CAD build for the part. Positions are in the model's coordinates, mm. A direction names the side the tool comes from. Coordinates: 2 decimals unless noted, no trailing zeros. Order: outer loops, then holes, each group sorted by start corner. A loop starts at its lowest first (then second) coordinate and runs counter-clockwise, first axis right, second up. Notation, with made-up numbers: (-6, 87.5) - (45, 87.5) arc R17 ccw to (45, 92.5) - close; hole circle Ø7 at (7, 53). An arc over 180 degrees is marked (long way). Write each question's results on one line, items separated by ' | '. Start each with the question number.
Q1. Band-saw the part on A-A, the plane z = -95. Write the cut outline in (x, y), then the cut area to 3 significant figures.
Q2. Band-saw the part on D-D, the plane x = -2.5. Write the cut outline in (y, z).
Q3. Pin check, flat tips, straight feed: P1, Ø10, axis at x = -25.5, y = 4.5, coming from the -Z side; P2, Ø4.5, axis at x = 1.5, y = 5.5, coming from the -Z side; P3, Ø1.5, axis at y = 10, z = -56.5, coming from the -X side. Stop position of each tip, or through.
Q4. Wall check: probe 1 along X at (y, z) = (19.75, -8.5); probe 2 along Z at (x, y) = (20, 3); probe 3 along Z at (x, y) = (3.5, 11.75). Give the ranges that are in metal, low to high.
Q5. Which spindle directions (+Z, -Z, +X, -X, +Y, -Y) get a long thin tool onto all of the face, cutting with end or side? Do faces 5 (the flat face through (-31.418, 10.846, -80.69)), 6 (the flat face through (-8.185, 10.846, -4.711)), 7 (the flat face through (17, 11, 0)). Say none if no direction does.
Q6. Pull direction X, two halves, no side cores. Call faces 1 (the flat face through (0, 0, -5)), 2 (the cylindrical face through (31.57, 10.85, -1.6)), 3 (the cylindrical face through (-25.38, 10.85, -115.85)), 4 (the flat face through (-30.812, 10.846, -60.328)): released by +X, released by -X, zero draft, split by the parting line, or undercut.
Q7. Band-saw the part on B-B, the plane x = 21. Write the cut outline in (y, z), then the cut area to 3 significant figures.
```python
from build123d import *

# Parameters (mm, degrees)
T_LE_DE_BASE_PLI_E1_DEPTH = 22
CONG_1_R                  = 2
BOSS_EXTRU_1_START        = -22
BOSS_EXTRU_1_DEPTH        = 22


# Sheet-metal steps are written as plain solids
with BuildPart() as part:
    # Esquisse1 → Tôle de base pliée1 (new body)
    with BuildSketch(Plane(origin=(0, 0, 0), x_dir=(1, 0, 0), z_dir=(0, 1, 0))):
        with BuildLine():
            Line((-16.269200028, 118.309493267), (-18.267296471, 118.396732042))
            ThreePointArc((-18.267296471, 118.396732042), (-25.459392421, 115.779023194), (-28.69397256, 108.842443699))
            Line((-28.69397256, 108.842443699), (-32.990482216, 10.436193874))
            ThreePointArc((-32.990482216, 10.436193874), (-30.223639621, 3.084869442), (-23, 0))
            Line((-23, 0), (-12, 0))
            ThreePointArc((-12, 0), (-10.279270691, 0.542543867), (-9.180922138, 1.97393957))
            Line((-9.180922138, 1.97393957), (-7.160115408, 7.52606043))
            ThreePointArc((-7.160115408, 7.52606043), (-6.061766854, 8.957456133), (-4.341037545, 9.5))
            Line((-4.341037545, 9.5), (4.341037545, 9.5))
            ThreePointArc((4.341037545, 9.5), (6.061766854, 8.957456133), (7.160115408, 7.52606043))
            Line((7.160115408, 7.52606043), (9.180922138, 1.97393957))
            ThreePointArc((9.180922138, 1.97393957), (10.279270691, 0.542543867), (12, 0))
            Line((12, 0), (23, 0))
            ThreePointArc((23, 0), (30.223639621, 3.084869442), (32.990482216, 10.436193874))
            Line((32.990482216, 10.436193874), (28.69397256, 108.842443699))
            ThreePointArc((28.69397256, 108.842443699), (25.459392421, 115.779023194), (18.267296471, 118.396732042))
            Line((18.267296471, 118.396732042), (16.269200028, 118.309493267))
            Line((16.269200028, 118.309493267), (16.22558064, 119.308541488))
            Line((16.22558064, 119.308541488), (18.223677083, 119.395780263))
            ThreePointArc((18.223677083, 119.395780263), (26.134982628, 116.516300531), (29.693020782, 108.886063087))
            Line((29.693020782, 108.886063087), (33.989530437, 10.479813261))
            ThreePointArc((33.989530437, 10.479813261), (30.946003583, 2.393356386), (23, -1))
            Line((23, -1), (12, -1))
            ThreePointArc((12, -1), (9.705694255, -0.276608177), (8.241229517, 1.631919427))
            Line((8.241229517, 1.631919427), (6.220422787, 7.184040287))
            ThreePointArc((6.220422787, 7.184040287), (5.488190418, 8.138304089), (4.341037545, 8.5))
            Line((4.341037545, 8.5), (-4.341037545, 8.5))
            ThreePointArc((-4.341037545, 8.5), (-5.488190418, 8.138304089), (-6.220422787, 7.184040287))
            Line((-6.220422787, 7.184040287), (-8.241229517, 1.631919427))
            ThreePointArc((-8.241229517, 1.631919427), (-9.705694255, -0.276608177), (-12, -1))
            Line((-12, -1), (-23, -1))
            ThreePointArc((-23, -1), (-30.946003583, 2.393356386), (-33.989530437, 10.479813261))
            Line((-33.989530437, 10.479813261), (-29.693020782, 108.886063087))
            ThreePointArc((-29.693020782, 108.886063087), (-26.134982628, 116.516300531), (-18.223677083, 119.395780263))
            Line((-18.223677083, 119.395780263), (-16.22558064, 119.308541488))
            Line((-16.22558064, 119.308541488), (-16.269200028, 118.309493267))
        make_face()
    extrude(amount=T_LE_DE_BASE_PLI_E1_DEPTH)

    # Congé1
    cong_1_edges = [part.edges().sort_by_distance(p)[0] for p in [
        (16.247390334, 22, -118.809017378),
        (16.247390334, 0, -118.809017378),
        (-16.247390334, 0, -118.809017378),
        (-16.247390334, 22, -118.809017378),
    ]]
    fillet(cong_1_edges, radius=CONG_1_R)

    # Esquisse2 → Boss.-Extru.1 (add)
    with BuildSketch(Plane(origin=(0, 22, 0), x_dir=(1, 0, 0), z_dir=(0, 1, 0)).offset(BOSS_EXTRU_1_START)):
        with BuildLine():
            Line((-29.693020782, 108.886063087), (-33.191022032, 51.694248192))
            Line((-33.191022032, 51.694248192), (-34.988578659, 10.523432648))
            ThreePointArc((-34.988578659, 10.523432648), (-31.668367545, 1.701843331), (-23, -2))
            Line((-23, -2), (23, -2))
            ThreePointArc((23, -2), (31.668367545, 1.701843331), (34.988578659, 10.523432648))
            Line((34.988578659, 10.523432648), (33.191022032, 51.694248192))
            Line((33.191022032, 51.694248192), (29.693020782, 108.886063087))
            Line((29.693020782, 108.886063087), (33.989530437, 10.479813261))
            ThreePointArc((33.989530437, 10.479813261), (30.946003583, 2.393356386), (23, -1))
            Line((23, -1), (12, -1))
            ThreePointArc((12, -1), (9.705694255, -0.276608177), (8.241229517, 1.631919427))
            Line((8.241229517, 1.631919427), (6.220422787, 7.184040287))
            ThreePointArc((6.220422787, 7.184040287), (5.488190418, 8.138304089), (4.341037545, 8.5))
            Line((4.341037545, 8.5), (-4.341037545, 8.5))
            ThreePointArc((-4.341037545, 8.5), (-5.488190418, 8.138304089), (-6.220422787, 7.184040287))
            Line((-6.220422787, 7.184040287), (-8.241229517, 1.631919427))
            ThreePointArc((-8.241229517, 1.631919427), (-9.705694255, -0.276608177), (-12, -1))
            Line((-12, -1), (-23, -1))
            ThreePointArc((-23, -1), (-30.946003583, 2.393356386), (-33.989530437, 10.479813261))
            Line((-33.989530437, 10.479813261), (-29.693020782, 108.886063087))
        make_face()
    extrude(amount=BOSS_EXTRU_1_DEPTH)


solid = part.part
```
Results below:
1) outline: (-30.54, 0) - (-29.3, 0) - (-29.3, 22) - (-30.54, 22) - close; (29.3, 0) - (30.54, 0) - (30.54, 22) - (29.3, 22) - close | area: 54.7 mm²
2) outline: (0, -9.5) - (22, -9.5) - (22, 2) - (0, 2) - close
3) P1: stops at z = -119.26 | P2: stops at z = -9.5 | P3: stops at x = -32.94
4) probe 1: x = -34.91 to -32.89, -6.58 to 6.58, 32.89 to 34.91 | probe 2: z = -119.33 to -118.32, 0 to 2 | probe 3: z = -9.5 to 2
5) face 5: -Z, -X, +Y, -Y | face 6: -Z, +Y, -Y | face 7: +Y, -Y
6) face 1: zero draft | face 2: released by +X | face 3: undercut | face 4: undercut
7) outline: (0, -119.16) - (22, -119.16) - (22, -118.14) - (0, -118.14) - close; (0, 0) - (22, 0) - (22, 2) - (0, 2) - close | area: 66.5 mm²
